```python
from build123d import *

# Parameters (mm, degrees)
F2_R     = 1.18745
F3_DEPTH = 4.572


with BuildPart() as f1:
    # F0 (on Front) → F1 (revolve)
    with BuildSketch(Plane.XZ):
        with BuildLine():
            Line((0, -4.203269), (0, 1.689531))
            Line((0, 1.689531), (-3.175, 1.001874))
            Line((-3.175, 1.001874), (-3.175, -1.030126))
            Line((-3.175, -1.030126), (-2.667, -1.030126))
            ThreePointArc((-2.667, -1.030126), (-1.834871, -1.822947), (-2.667, -2.615769))
            ThreePointArc((-2.667, -2.615769), (-3.46075, -3.409519), (-2.667, -4.203269))
            Line((-2.667, -4.203269), (0, -4.203269))
        make_face()
    revolve(axis=Axis((0, 0, 0.38379), (0, 0, -1)))

    # F2 (on face) → F3 (cut)
    with BuildSketch(Plane(origin=(0, 0, -4.203269), x_dir=(1, 0, 0), z_dir=(0, 0, -1))):
        Circle(F2_R)
    extrude(amount=-F3_DEPTH, mode=Mode.SUBTRACT)


solid = f1.part
```
Design review of the part built by this model. Coordinates are the model's own, in mm. A direction names the side the tool comes from. Coordinates: 2 decimals unless noted, no trailing zeros. Order: outer loops, then holes, each group sorted by start corner. A loop starts at its lowest first (then second) coordinate and runs counter-clockwise, first axis right, second up. Notation, with made-up numbers: (-19, -19) -> (39, -19) arc R5 ccw to (39, -13) -> close; hole circle Ø6 at (88.25, -18.5). An arc over 180 degrees is marked (long way). One line per item, written item: value. Start each with the question number.
Q1. Insertion check: pin 1 Ø0.7 at (x, y) = (0.5, 0) entering from -Z; pin 2 Ø1.5 at (x, y) = (-0.5, 1) entering from +Z; pin 3 Ø1 at (x, z) = (1.5, -3.5) entering from -Y. Each pin has a flat end and moves straight along its axis. Give the tip position at first contact, or say it passes through.
Q2. Mouldability with a two-part tool opening along Y and no side actions: class faces 1 (the flat face through (2, 2, -1.03)), 2 (the flat face through (0, 0, 0.369)), 3 (the conical face through (0.043, -0.194, 1.647)) as pulls with the +Y half, pulls with the -Y half, needs draft (parallel to the pull), parting line crosses it, or undercut.
Q3. For probe 1 along X at (y, z) = (-1, -1.9); probe 2 along Z at (x, y) = (2.5, -1.25); probe 3 along X at (y, z) = (0, -1.35), list the stretches that pass through material, from the lowest coordinate up.
Q4. Take a section at A-A, the plane z = 0.2. State the section outline as (x, y) points (3 decimals).
Q5. Tool access review of faces 4 (the cylindrical face through (-0.88, -0.8, -1.95)), 5 (the flat face through (-1, -1, -4.203)), 6 (the cylindrical face through (0.69, -3.1, -0.03)): name each direction out of +Z, -Z, +X, -X, +Y, -Y from which nothing blocks a thin tool from reaching the whole face with its end or side.
Values follow:
1. pin 1: stops at z = 0.37
1. pin 2: stops at z = 1.61
1. pin 3: stops at y = -3.31
2. face 1: needs draft
2. face 2: undercut
2. face 3: parting line crosses it
3. probe 1: x = -1.54 to -0.64, 0.64 to 1.54
3. probe 2: z = -4.19 to -2.63, -1.03 to 1.08
3. probe 3: x = -1.99 to -1.19, 1.19 to 1.99
4. outline: circle Ø6.35 at (0, 0); hole circle Ø2.375 at (0, 0)
5. face 4: -Z
5. face 5: -Z, +X, -X, +Y, -Y
5. face 6: +Z
